from build123d import *

# Parameters (mm, degrees)
BOSS_EXTRUDE1_DEPTH        = 1.4
F_2_5_2_5_DIAMETER_SLOT1_D = 2.5
BOSS_EXTRUDE2_DEPTH        = 2
BOSS_EXTRUDE3_DEPTH        = 3
SKETCH8_W                  = 0.8
SKETCH8_H                  = 0.8
BOSS_EXTRUDE4_DEPTH        = 2
SKETCH9_W                  = 0.8
SKETCH9_H                  = 0.8
BOSS_EXTRUDE5_DEPTH        = 8
LPATTERN1_COUNT            = 6
LPATTERN1_PITCH            = 2.62
FILLET1_R                  = 0.4


with BuildPart() as part:
    # Sketch1 → Boss-Extrude1 (new body)
    with BuildSketch(Plane.XY):
        Polygon((-17.623529412, 12), (-16.623529412, 13), (23.376470588, 13), (24.376470588, 12), (24.376470588, -10), (23.376470588, -11), (-17.623529412, -11), (-17.623529412, 0), (-16.823529412, 0), (-16.823529412, 5), (-17.623529412, 5), align=None)
    extrude(amount=BOSS_EXTRUDE1_DEPTH)

    # Ø2.5 (2.5) Diameter Slot1 (through all)
    with Locations(Plane.XY.offset(1.4)):
        with Locations((-15.874285672, -9.269193445), (-15.874285672, 11.312714255), (22.710754066, -9.269193445), (22.710754066, 11.312714255)):
            Hole(F_2_5_2_5_DIAMETER_SLOT1_D / 2)

    # Sketch6 → Boss-Extrude2 (add)
    with BuildSketch(Plane.XY.offset(1.4)):
        Polygon((-15.083529412, -6.7), (-0.083529412, -6.7), (-0.083529412, 8.3), (-14.083529412, 8.3), (-14.083529412, -1.2), (-15.083529412, -3.2), align=None)
    extrude(amount=BOSS_EXTRUDE2_DEPTH)

    # Sketch7 → Boss-Extrude3 (add)
    with BuildSketch(Plane.XY.offset(1.4)):
        with BuildLine():
            Line((22.126470588, 6.1), (22.126470588, 5.6))
            ThreePointArc((22.126470588, 5.6), (22.303247284, 5.526776695), (22.376470588, 5.35))
            Line((22.376470588, 5.35), (22.376470588, 3.78))
            ThreePointArc((22.376470588, 3.78), (22.303247284, 3.603223305), (22.126470588, 3.53))
            Line((22.126470588, 3.53), (22.126470588, 3.03))
            ThreePointArc((22.126470588, 3.03), (22.303247284, 2.956776695), (22.376470588, 2.78))
            Line((22.376470588, 2.78), (22.376470588, 1.21))
            ThreePointArc((22.376470588, 1.21), (22.303247284, 1.033223305), (22.126470588, 0.96))
            Line((22.126470588, 0.96), (22.126470588, 0.46))
            ThreePointArc((22.126470588, 0.46), (22.303247284, 0.386776695), (22.376470588, 0.21))
            Line((22.376470588, 0.21), (22.376470588, -1.36))
            ThreePointArc((22.376470588, -1.36), (22.303247284, -1.536776695), (22.126470588, -1.61))
            Line((22.126470588, -1.61), (22.126470588, -2.11))
            ThreePointArc((22.126470588, -2.11), (22.303247284, -2.183223305), (22.376470588, -2.36))
            Line((22.376470588, -2.36), (22.376470588, -3.93))
            ThreePointArc((22.376470588, -3.93), (22.303247284, -4.106776695), (22.126470588, -4.18))
            Line((22.126470588, -4.18), (22.126470588, -4.68))
            ThreePointArc((22.126470588, -4.68), (22.303247284, -4.753223305), (22.376470588, -4.93))
            Line((22.376470588, -4.93), (22.376470588, -6.75))
            ThreePointArc((22.376470588, -6.75), (22.303247284, -6.926776695), (22.126470588, -7))
            Line((22.126470588, -7), (19.626470588, -7))
            ThreePointArc((19.626470588, -7), (19.449693893, -6.926776695), (19.376470588, -6.75))
            Line((19.376470588, -6.75), (19.376470588, -4.93))
            ThreePointArc((19.376470588, -4.93), (19.449693893, -4.753223305), (19.626470588, -4.68))
            Line((19.626470588, -4.68), (19.626470588, -4.18))
            ThreePointArc((19.626470588, -4.18), (19.449693893, -4.106776695), (19.376470588, -3.93))
            Line((19.376470588, -3.93), (19.376470588, -2.36))
            ThreePointArc((19.376470588, -2.36), (19.449693893, -2.183223305), (19.626470588, -2.11))
            Line((19.626470588, -2.11), (19.626470588, -1.61))
            ThreePointArc((19.626470588, -1.61), (19.449693893, -1.536776695), (19.376470588, -1.36))
            Line((19.376470588, -1.36), (19.376470588, 0.21))
            ThreePointArc((19.376470588, 0.21), (19.449693893, 0.386776695), (19.626470588, 0.46))
            Line((19.626470588, 0.46), (19.626470588, 0.96))
            ThreePointArc((19.626470588, 0.96), (19.449693893, 1.033223305), (19.376470588, 1.21))
            Line((19.376470588, 1.21), (19.376470588, 2.78))
            ThreePointArc((19.376470588, 2.78), (19.449693893, 2.956776695), (19.626470588, 3.03))
            Line((19.626470588, 3.03), (19.626470588, 3.53))
            ThreePointArc((19.626470588, 3.53), (19.449693893, 3.603223305), (19.376470588, 3.78))
            Line((19.376470588, 3.78), (19.376470588, 5.35))
            ThreePointArc((19.376470588, 5.35), (19.449693893, 5.526776695), (19.626470588, 5.6))
            Line((19.626470588, 5.6), (19.626470588, 6.1))
            ThreePointArc((19.626470588, 6.1), (19.449693893, 6.173223305), (19.376470588, 6.35))
            Line((19.376470588, 6.35), (19.376470588, 8.17))
            ThreePointArc((19.376470588, 8.17), (19.449693893, 8.346776695), (19.626470588, 8.42))
            Line((19.626470588, 8.42), (22.126470588, 8.42))
            ThreePointArc((22.126470588, 8.42), (22.303247284, 8.346776695), (22.376470588, 8.17))
            Line((22.376470588, 8.17), (22.376470588, 6.35))
            ThreePointArc((22.376470588, 6.35), (22.303247284, 6.173223305), (22.126470588, 6.1))
        make_face()
    extrude(amount=BOSS_EXTRUDE3_DEPTH)

    # Sketch8 → Boss-Extrude4 (add)
    with BuildSketch(Plane.XY.offset(4.4)):
        with Locations((20.876470588, -5.84)):
            Rectangle(SKETCH8_W, SKETCH8_H)
        with Locations((20.876470588, -3.22)):
            Rectangle(SKETCH8_W, SKETCH8_H)
        with Locations((20.876470588, -0.6)):
            Rectangle(SKETCH8_W, SKETCH8_H)
        with Locations((20.876470588, 2.02)):
            Rectangle(SKETCH8_W, SKETCH8_H)
        with Locations((20.876470588, 4.64)):
            Rectangle(SKETCH8_W, SKETCH8_H)
        with Locations((20.876470588, 7.26)):
            Rectangle(SKETCH8_W, SKETCH8_H)
    extrude(amount=BOSS_EXTRUDE4_DEPTH)

    # Sketch9 → Boss-Extrude5 (add)
    with BuildSketch(Plane(origin=(21.276470588, 0, 0), x_dir=(0, 0, -1), z_dir=(1, 0, 0))):
        with Locations((-6, 7.26)):
            Rectangle(SKETCH9_W, SKETCH9_H)
    boss_extrude5 = extrude(amount=BOSS_EXTRUDE5_DEPTH)

    # LPattern1: Boss-Extrude5 ×6
    with Locations(*[(0, -i * LPATTERN1_PITCH, 0) for i in range(1, LPATTERN1_COUNT)]):
        add(boss_extrude5)

    # Fillet1
    fillet1_edges = [part.edges().sort_by_distance(p)[0] for p in [
        (20.476470588, -5.84, 6.4),
        (20.476470588, -3.22, 6.4),
        (20.476470588, -0.6, 6.4),
        (20.476470588, 2.02, 6.4),
        (20.476470588, 4.64, 6.4),
        (20.476470588, 7.26, 6.4),
    ]]
    fillet(fillet1_edges, radius=FILLET1_R)


solid = part.part
Can you work these out from the model? Positions are in its coordinate system, mm. A direction names the side the tool comes from. Round coordinates to 2 decimals unless told otherwise and drop trailing zeros. Order: outer loops, then holes, each group sorted by start corner. A loop starts at its lowest first (then second) coordinate and runs counter-clockwise, first axis right, second up. Notation, with made-up numbers: M 13.5,17 L 32.5,17 A3 cw 32.5,22 Z; hole C 79,28.5 d11. An arc over 180 degrees is marked long. Use a Markdown table: item, result.
1) If we mould it in two halves opening along Y, with no side actions, what happens to faces 6 (the face through (25, -0.2, 6)), 7 (the face through (-8, -6.7, 2)), 8 (the face through (24.376, 1, 1))? For each: +Y half, -Y half, draft (parallel to the pull), parting line (faces both ways), or undercut.
Geometry says:
| item | result |
|---|---|
| face 6 | undercut |
| face 7 | -Y half |
| face 8 | draft |
2) I'm going to push flat-ended pins straight in: P1, Ø0.8, axis at x = 21, z = 3, coming from the +Y side; P2, Ø1, axis at y = 6, z = 5.5, coming from the +X side; P3, Ø1.6, axis at x = 23, z = 5, coming from the -Y side; P4, Ø1.7, axis at y = 4.5, z = 3, coming from the +X side. Where does each tip first touch, or does it pass through?
Geometry says:
| item | result |
|---|---|
| P1 | stops at y = 8.42 |
| P2 | passes through |
| P3 | stops at y = -6.24 |
| P4 | stops at x = 22.38 |
3) On a 3-axis mill with a long thin cutter (end or side, diameter ignored), from which of +Z, -Z, +X, -X, +Y, -Y can I reach the whole of each face in a straight line? I mean faces 1 (the face through (-16.546, -8.215, 0.69)), 2 (the face through (21, 8.42, 3)), 3 (the face through (21.276, 7.3, 5)), 4 (the face through (25, 5.04, 6)), 5 (the face through (-0.084, 1, 2)). Say none if no direction works.
Geometry says:
| item | result |
|---|---|
| face 1 | +Z, -Z |
| face 2 | +Z, +X, -X, +Y |
| face 3 | +X, +Y, -Y |
| face 4 | +Z, +X, -X |
| face 5 | +Z, +Y, -Y |
4) If I drill on line 1 along Y through (x, z) = (25.5, 6.25); line 2 along X through (y, z) = (-0.25, 2.5); line 3 along X through (y, z) = (-5.25, 1.5), over which ranges is the centre line in solid material (lowest first)?
Geometry says:
| item | result |
|---|---|
| line 1 | y = -6.24 to -5.44, -3.62 to -2.82, -1 to -0.2, 1.62 to 2.42, 4.24 to 5.04, 6.86 to 7.66 |
| line 2 | x = -14.08 to -0.08, 19.38 to 22.38 |
| line 3 | x = -15.08 to -0.08, 19.38 to 22.38 |
5) Imagine slicing it at C-C (x = -11.5). List the corners of the cut face in (y, z) for me, then the cut area to 3 significant figures.
Geometry says:
| item | result |
|---|---|
| outline | M -11,0 L 13,0 L 13,1.4 L 8.3,1.4 L 8.3,3.4 L -6.7,3.4 L -6.7,1.4 L -11,1.4 Z |
| area | 63.6 mm² |
6) Imagine slicing it at D-D (x = 5). List the corners of the cut face in (y, z) for me.
Geometry says:
| item | result |
|---|---|
| outline | M -11,0 L 13,0 L 13,1.4 L -11,1.4 Z |
7) Imagine slicing it at A-A (x = 25). List the corners of the cut face in (y, z) for me.
Geometry says:
| item | result |
|---|---|
| outline | M -6.24,5.6 L -5.44,5.6 L -5.44,6.4 L -6.24,6.4 Z; M -3.62,5.6 L -2.82,5.6 L -2.82,6.4 L -3.62,6.4 Z; M -1,5.6 L -0.2,5.6 L -0.2,6.4 L -1,6.4 Z; M 1.62,5.6 L 2.42,5.6 L 2.42,6.4 L 1.62,6.4 Z; M 4.24,5.6 L 5.04,5.6 L 5.04,6.4 L 4.24,6.4 Z; M 6.86,5.6 L 7.66,5.6 L 7.66,6.4 L 6.86,6.4 Z |
8) Imagine slicing it at B-B (z = 5). List the corners of the cut face in (x, y) for me.
Geometry says:
| item | result |
|---|---|
| outline | M 20.48,-6.24 L 21.28,-6.24 L 21.28,-5.44 L 20.48,-5.44 Z; M 20.48,-3.62 L 21.28,-3.62 L 21.28,-2.82 L 20.48,-2.82 Z; M 20.48,-1 L 21.28,-1 L 21.28,-0.2 L 20.48,-0.2 Z; M 20.48,1.62 L 21.28,1.62 L 21.28,2.42 L 20.48,2.42 Z; M 20.48,4.24 L 21.28,4.24 L 21.28,5.04 L 20.48,5.04 Z; M 20.48,6.86 L 21.28,6.86 L 21.28,7.66 L 20.48,7.66 Z |
